```python
from build123d import *

# Parameters (mm, degrees)
F0_R     = 49.5
F1_DEPTH = 24
F2_R     = 43
F3_DEPTH = 3
F4_R     = 36.5
F5_DEPTH = 3


with BuildPart() as f1:
    # F0 (on Right) → F1 (new body)
    with BuildSketch(Plane.YZ):
        with Locations((-14.71213, 24.086773)):
            Circle(F0_R)
    extrude(amount=F1_DEPTH)

    # F2 (on face) → F3 (cut)
    with BuildSketch(Plane.YZ.offset(24)):
        with Locations((-14.71213, 24.086773)):
            Circle(F2_R)
    extrude(amount=-F3_DEPTH, mode=Mode.SUBTRACT)

    # F4 (on face) → F5 (cut)
    with BuildSketch(Plane(origin=(0, 0, 0), x_dir=(0, -1, 0), z_dir=(-1, 0, 0))):
        with Locations((14.71213, 24.086773)):
            Circle(F4_R)
    extrude(amount=-F5_DEPTH, mode=Mode.SUBTRACT)


solid = f1.part
```
Check sheet for the modelled part. Datum: model origin and axes. Units: mm. A direction names the side the tool comes from. Round coordinates to 2 decimals unless told otherwise and drop trailing zeros. Loops run counter-clockwise (first coordinate to the right, second up) from the corner with the lowest first, then second, coordinate; pieces in that order, holes last. Notation, with made-up numbers: (-17.75, 8.25) -> (-1.75, 8.25) arc R10 cw to (-1.75, 18.25) -> close; hole circle Ø2 at (67.25, 16). An arc over 180 degrees is marked (long way). Write item = value, one per line. Start each with the question number.
1) Sectioned sample at D-D, the plane y = -17. Record the cut outline in (x, z) (3 decimals).
2) Sectioned sample at C-C, the plane x = 22.5. Record the cut outline in (y, z), plus the area to 3 significant figures.
3) Release check for a two-part mould opening along Y. For faces 1 (the flat face through (21, -15, 25)), 2 (the cylindrical face through (11.832, -25.443, -24.236)), 3 (the flat face through (24, -30, 65)) record: released by +Y, released by -Y, zero draft, split by the parting line, or undercut.
4) Thickness scan on probe 1 along X at (y, z) = (-20, 44); probe 2 along Z at (x, y) = (8.25, -15.5); probe 3 along Z at (x, y) = (21.5, 21.5). Record the ranges inside material, lowest first.
5) Gauge pin test, flat ends, axial feed: pin 1 Ø12 at (x, y) = (21, -53.5) entering from -Z; pin 2 Ø10 at (y, z) = (7, 18.5) entering from -X; pin 3 Ø4 at (x, y) = (14.5, -26.5) entering from +Z. Record the tip position at first contact, or that the pin passes through.
6) Sectioned sample at B-B, the plane y = 23. Record the cut outline in (x, z), plus the area to 3 significant figures.
7) Sectioned sample at A-A, the plane z = 53.5. Record the cut outline in (x, y), plus the area to 3 significant figures.
8) Set-up check for faces 4 (the cylindrical face through (1.479, -6.8, -11.545)), 5 (the flat face through (0, -33, -9)), 6 (the cylindrical face through (22.521, 26.302, 37.003)): record each of +Z, -Z, +X, -X, +Y, -Y from which the full face is reachable in a straight line by a thin tool's end or side.
Results are:
q1.outline = (0, -25.36) -> (24, -25.36) -> (24, -18.852) -> (21, -18.852) -> (21, 67.026) -> (24, 67.026) -> (24, 73.534) -> (0, 73.534) -> (0, 60.515) -> (3, 60.515) -> (3, -12.341) -> (0, -12.341) -> close
q2.outline = circle Ø99 at (-14.71, 24.09); hole circle Ø86 at (-14.71, 24.09)
q2.area = 1,890 mm^2
q3.face_1 = undercut
q3.face_2 = split by the parting line
q3.face_3 = zero draft
q4.probe_1 = 3 to 21
q4.probe_2 = -25.41 to 73.58
q4.probe_3 = -9.66 to 0.9, 47.27 to 57.83
q5.pin_1 = -13
q5.pin_2 = 3
q5.pin_3 = 72.61
q6.outline = (0, -7.98) -> (24, -7.98) -> (24, 3.43) -> (21, 3.43) -> (21, 44.75) -> (24, 44.75) -> (24, 56.15) -> (0, 56.15) -> close
q6.area = 1,420 mm^2
q7.outline = (0, -54.53) -> (24, -54.53) -> (24, -46.08) -> (21, -46.08) -> (21, 16.65) -> (24, 16.65) -> (24, 25.1) -> (0, 25.1) -> (0, 6.9) -> (3, 6.9) -> (3, -36.32) -> (0, -36.32) -> close
q7.area = 1,590 mm^2
q8.face_4 = -X
q8.face_5 = +Z, -Z, -X, +Y, -Y
q8.face_6 = +X
